Check sheet for the modelled part. Datum: model origin and axes. Units: mm. A direction names the side the tool comes from. Round coordinates to 2 decimals unless told otherwise and drop trailing zeros. Loops run counter-clockwise (first coordinate to the right, second up) from the corner with the lowest first, then second, coordinate; pieces in that order, holes last. Notation, with made-up numbers: (-11, -30.75) - (35, -30.75) arc R20 ccw to (35, -11.75) - close; hole circle Ø10 at (89, -34.75). An arc over 180 degrees is marked (long way). Put each result on its own line as item: value.
Autodesk Inventor part; units mm, degrees
ref_plane "YZ Plane" through (0, 0, 0) normal (1, 0, 0) x (0, 1, 0)
ref_plane "XZ Plane" through (0, 0, 0) normal (0, 1, 0) x (-1, 0, 0)
ref_plane "XY Plane" through (0, 0, 0) normal (0, 0, 1) x (1, 0, 0)
sketch "Sketch1" plane through (0, 0, 0) normal (0, 0, 1) x (1, 0, 0)
  line L0 (0, 0) -> (-50, 0)
  line L1 (-50, 0) -> (-50, 50)
  line L2 (-50, 50) -> (0, 50)
  line L3 (0, 50) -> (0, 0)
  dimension "d0" = 50
  dimension "d1" = 50
extrude "Extrusion1" add sketch "Sketch1" along normal blind 10
sketch "Sketch2" plane through (0, 0, 10) normal (0, 0, 1) x (1, 0, 0)
  line L0 (-49.9965, 0) -> (0.0035, 0)
  line L1 (0.0035, 0) -> (0.0035, 10)
  line L2 (0.0035, 10) -> (-49.9965, 10)
  line L3 (-49.9965, 10) -> (-49.9965, 0)
  point P0 (0, 0)
  dimension "d4" = 50
  dimension "d5" = 10
extrude "Extrusion2" add sketch "Sketch2" along normal blind 30
fillet "Fillet3" radius 5 6 edges at (-49.9965, 10, 25) (0.0035, 10, 25) (0, 30, 10) (-50, 25, 10) (-50, 25, 0) (0, 25, 0)
fillet "Fillet5" radius 5 11 edges at (-1.4609, 8.5355, 40) (-24.9965, 10, 40) (-48.532, 8.5355, 40) (-49.9965, 2.5, 40) (0.0035, 2.5, 40) (-1.4644, 50, 8.5356) (-48.5356, 50, 8.5356) (-1.4645, 50, 1.4645) (-48.5355, 50, 1.4645) (-25, 50, 0) (-25, 50, 10)
properties part number "Marker Holder 90 deg"
Item 1: Tool access check on faces 1 (the cylindrical face through (-1.422, 2.465, 38.496)), 2 (the cylindrical face through (-1.422, 8.496, 20.21)), 3 (the flat face through (-25, 28, 10)). Record the directions out of +Z, -Z, +X, -X, +Y, -Y that give a thin tool (end or side, any length) a straight path to the whole face; none if there is none.
Filled sheet:
face 1: +Z, +X, +Y, -Y
face 2: +Z, +X, +Y
face 3: +Z, +X, -X, +Y
Item 2: Section check D-D on z = 9. Enter the section's corners in (x, y), then the cut area to 3 significant figures.
Filled sheet:
outline: (-50, 0) - (0, 0) - (0, 5.19) arc R5 ccw to (-2, 9) - (-2, 45) arc R3 ccw to (-5, 48) - (-45, 48) arc R3 ccw to (-48, 45) - (-48, 9) arc R5 ccw to (-50, 5) - close
area: 2,240 mm²
Item 3: Section check B-B on z = 23. Enter the section's corners in (x, y).
Filled sheet:
outline: (-50, 0) - (0, 0) - (0, 5) arc R5 ccw to (-5, 10) - (-45, 10) arc R5 ccw to (-50, 5) - close
Item 4: Go/stop test with flat-tipped pins: pin 1 (10 mm diameter, centred on x = -28, z = 12, fed in from +Y); pin 2 (2 mm diameter, centred on x = -36.5, z = 14.5, fed in from +Y); pin 3 (5.5 mm diameter, centred on y = 13.5, z = 8, fed in from +X). Record where each tip stops, or that it passes through.
Filled sheet:
pin 1: y = 49.58
pin 2: y = 10
pin 3: x = -0.01
Item 5: Thickness scan on line 1 (Z direction, x = -39, y = 42.5); line 2 (Z direction, x = -7.5, y = 9). Record the ranges inside material, lowest first. Write a range as from..to.
Filled sheet:
line 1: 0..10
line 2: 0..38
